Autodesk Inventor part; units mm, degrees
ref_plane "YZ Plane" through (0, 0, 0) normal (1, 0, 0) x (0, 1, 0)
ref_plane "XZ Plane" through (0, 0, 0) normal (0, 1, 0) x (-1, 0, 0)
ref_plane "XY Plane" through (0, 0, 0) normal (0, 0, 1) x (1, 0, 0)
sketch "スケッチ1" plane through (0, 0, 0) normal (1, 0, 0) x (0, 1, 0)
  circle A0 centre (-4.4971, 26.9328) radius 3.6
  circle A1 centre (-4.4971, 26.9328) radius 3
  arc A2 (1.1321, 30.1828) -> (-10.1263, 23.6828) centre (-4.4971, 26.9328) ccw
  line L0 (-10.1263, 23.6828) -> (-8.4019, 20.6962)
  line L1 (-8, 19.1962) -> (-8, 0)
  line L2 (8, 0) -> (8, 17.7513)
  line L3 (7.7321, 18.7513) -> (1.1321, 30.1828)
  arc A3 (8, 17.7513) -> (7.7321, 18.7513) centre (6, 17.7513) ccw
  arc A4 (-8, 0) -> (8, 0) centre (0, 0) ccw
  circle A5 centre (0, 0) radius 2
  line L4 (-8, 20) -> (-8, 0) construction
  line L5 (-8, 0) -> (0, 0) construction
  line L6 (0, -28.9489) -> (0, 46.6055) construction
  arc A6 (-8, 19.1962) -> (-8.4019, 20.6962) centre (-11, 19.1962) ccw
  circle A7 centre (8.75, -15.1554) radius 3
  line L7 (0, 0) -> (8.75, -15.1554) construction
  circle A8 centre (0, 0) radius 8 construction
  line L8 (-5.4965, -5.8127) -> (6.6888, -17.3352)
  line L9 (11.6683, -14.4603) -> (7.7823, 1.8538)
  circle A9 centre (8.75, -15.1554) radius 2
  circle A10 centre (8.75, -15.1554) radius 1
  circle A11 centre (-4.4971, 26.9328) radius 5.5 construction
  line L10 (0.9991, 27.1358) -> (1.9986, 0.0738) construction
  line L11 (-9.7612, 25.3391) -> (-1.9142, -0.5795) construction
  point P0 (8, 18.2872)
  point P1 (8, 0.9397)
  point P2 (-5.4965, -5.8127)
  dimension "d0" = 6
  dimension "d1" = 7.2
  dimension "d2" = 6.5
  dimension "d9" = 2
  dimension "d13" = 150
  dimension "d14" = 8
  dimension "d15" = 4
  dimension "d18" = 13.2
  dimension "d19" = 8
  dimension "d20" = 20
  dimension "d26" = 3
  dimension "d55" = 6
  dimension "d56" = 17.5
  dimension "d58" = 30
  dimension "d59" = 16
  dimension "d60" = 4
  dimension "d61" = 2
  dimension "d75" = 11
extrude "押し出し3" add sketch "スケッチ1" along normal blind 2.5 contours A0 | L3 A3 L2 A4 L1 A6 L0 A2 | L9 A7 L8 A4 L2 | A7 | A5
sketch "スケッチ2" plane through (2.5, 0, 0) normal (1, 0, 0) x (0, 0, -1)
  line L0 (-0.9397, 8) -> (-17.7513, 8)
  arc A0 (-17.7513, 8) -> (-18.7513, 7.7321) centre (-17.7513, 6) ccw
  line L1 (-18.7513, 7.7321) -> (-30.1828, 1.1321)
  arc A1 (-30.1828, 1.1321) -> (-23.6828, -10.1263) centre (-26.9328, -4.4971) ccw
  line L2 (-23.6828, -10.1263) -> (-20.6962, -8.4019)
  arc A2 (-19.1962, -8) -> (-20.6962, -8.4019) centre (-19.1962, -11) ccw
  line L3 (-19.1962, -8) -> (0, -8)
  arc A3 (0, -8) -> (5.8127, -5.4965) centre (0, 0) ccw
  circle A4 centre (-26.9328, -4.4971) radius 3.6
  line L4 (5.8127, -5.4965) -> (17.3352, 6.6888)
  arc A5 (17.3352, 6.6888) -> (14.4603, 11.6683) centre (15.1554, 8.75) ccw
  line L5 (14.4603, 11.6683) -> (-0.9397, 8)
  dimension "d32" = 7.2
extrude "押し出し4" cut sketch "スケッチ2" against normal blind 0.6 contours A4
extrude "押し出し5" add sketch "スケッチ1" along normal blind 1.5 contours A9
properties part number "GearCover"
The listing builds one solid part. Answer for the finished solid, in the listing's coordinates (mm). A direction names the side the tool comes from. Coordinates: 2 decimals unless noted, no trailing zeros. Loops run counter-clockwise (first coordinate to the right, second up) from the corner with the lowest first, then second, coordinate; pieces in that order, holes last. Notation, with made-up numbers: M 14.25,86 L 63.25,86 A9 ccw 63.25,94 Z; hole C 86.25,76 d4. An arc over 180 degrees is marked long. Answer as a JSON object with one key per item and string values. Group by question number.
Item 1: Section A-A (z = 29) is taken. Write down the section's boundary in (x, y) (3 decimals).
Item 2: Section D-D (z = 5) is taken. Write down the section's boundary in (x, y), and give its area (3 significant figures).
Item 3: Which of the six approach directions +Z, -Z, +X, -X, +Y, -Y give full straight-line access (tool end or side, diameter ignored) to faces 5 (the face through (1.23, -7.87, 32.49)), 6 (the face through (1, 8, 9)), 7 (the face through (2.2, -4.34, 30.53)), 8 (the face through (0, 0, 8)), 9 (the face through (1, -8, 10))?
Item 4: Section C-C (x = 0.75) is taken. Write down the section's boundary in (y, z), and give its area (3 significant figures).
Item 5: Each of these flat-tipped pins is pushed along its axis until it touches: P1, Ø3, axis at y = 8, z = -15, coming from the +X side; P2, Ø1, axis at x = 2, y = -3, coming from the -Z side; P3, Ø0.8, axis at x = 1, z = 9.5, coming from the -Y side; P4, Ø1, axis at x = 1, y = 4, coming from the +Z side. Where does it stop, or does it pass through?
Item 6: Section B-B (y = -7) is taken. Write down the section's boundary in (x, z).
Item 7: Consider L1, parallel to Y at x = 1.15, z = 17; L2, parallel to Z at x = 1.4, y = -3.25; L3, parallel to Z at x = 1.4, y = -4.5 (3 decimals). Determine where each line is inside the solid, lowest interval first.
Item 8: Determine the mould class of faces 1 (the face through (1.5, 9, -14)), 2 (the face through (1.232, -9.276, 22.21)), 3 (the face through (1.232, 10.296, -17.726)), 4 (the face through (2.5, 0, 8)) for opening direction Y: +Y half, -Y half, draft (parallel to the pull), parting line (faces both ways), or undercut.
Solved:
{
 "1": {"outline": "M 0,-10.66 L 2.5,-10.66 L 2.5,-7.444 L 1.9,-7.444 L 1.9,-6.671 L 0,-6.671 Z; M 0,-2.323 L 1.9,-2.323 L 1.9,-1.55 L 2.5,-1.55 L 2.5,1.815 L 0,1.815 Z"},
 "2": {"outline": "M 0,-8 L 2.5,-8 L 2.5,8 L 0,8 Z", "area": "40.0 mm2"},
 "3": {"face 5": "+X, -X", "face 6": "+Z, +X, -X, +Y", "face 7": "+X", "face 8": "+Z, -Z, -X, +Y, -Y", "face 9": "-Z, +X, -X, -Y"},
 "4": {"outline": "M -10.13,23.68 L -8.4,20.7 A3 cw -8,19.2 L -8,0 A8 ccw -5.5,-5.81 L 6.69,-17.34 A3 ccw 11.67,-14.46 L 8,0.94 L 8,17.75 A2 ccw 7.73,18.75 L 1.13,30.18 A6.5 ccw Z; hole C -4.5,26.93 d6; hole C 8.75,-15.16 d2", "area": "673 mm2"},
 "5": {"P1": "stops at x = 2.5", "P2": "stops at z = -8.65", "P3": "stops at y = -8", "P4": "stops at z = 26.08"},
 "6": {"outline": "M 0,-3.87 L 2.5,-3.87 L 2.5,24.35 L 1.9,24.35 L 1.9,25.28 L 0,25.28 Z; M 0,28.59 L 1.9,28.59 L 1.9,29.52 L 2.5,29.52 L 2.5,32.93 L 0,32.93 Z"},
 "7": {"L1": "y = -8 to 8", "L2": "z = -7.94 to 24.2, 29.66 to 33.31", "L3": "z = -6.755 to 23.933, 29.933 to 33.433"},
 "8": {"face 1": "undercut", "face 2": "-Y half", "face 3": "parting line", "face 4": "draft"}
}
